Drawing for the job (mm, zero at the part's lowest x, y, z). Give positions to 0.01 mm unless a question says otherwise; leave off trailing zeros. Loops run counter-clockwise (first coordinate to the right, second up) from the corner with the lowest first, then second, coordinate; pieces in that order, holes last. Notation, with made-up numbers: (58, -8.75) -> (64, -8.75) arc R17 ccw to (64, 14.25) -> close; hole circle Ø4 at (44, 58). An arc over 180 degrees is marked (long way). Use CSV: the item, a comma, the result in double quotes. Start each with the question number.
(1) Cut at A-A on y = 5. Write the cut outline in (x, z).
(2) Flat gauge pins, fed straight in: pin 1 (1 mm diameter, centred on x = 33, y = 20, fed in from +Z); pin 2 (5 mm diameter, centred on y = 30, z = 51, fed in from +X); pin 3 (8 mm diameter, centred on y = 22, z = 18, fed in from +X). Where does each tip first touch, or does it go through?
(3) Pull direction Z, two halves, no side cores. Call the marked faces 1, 2, 3 and 4: pulls with the +Z half, pulls with the -Z half, needs draft (parallel to the pull), parting line crosses it, or undercut.
(4) Cut at C-C on z = 36. Write the cut outline in (x, y).
(5) Cut at B-B on x = 36. Write the cut outline in (y, z).
(6) Drill centre lines: probe 1 along Z at (x, y) = (35, 19); probe 2 along Z at (x, y) = (60, 4); probe 3 along X at (y, z) = (30.5, 52.5). Where is each one in solid material? Low to high.
(7) Cut at D-D on y = 26. Write the cut outline in (x, z).
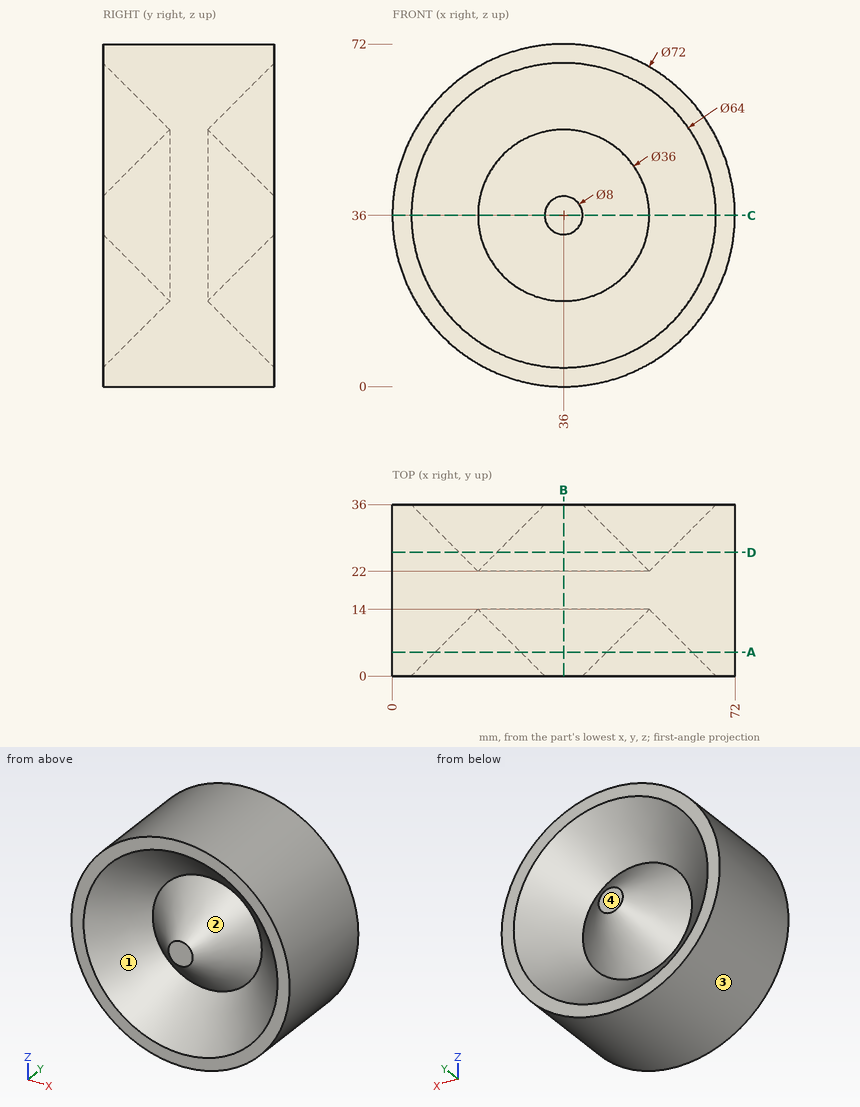
Check result:
1,outline,"circle Ø72 at (36, 36); circle Ø18 at (36, 36); hole circle Ø54 at (36, 36)"
2,pin 1,"z = 71.91"
2,pin 2,"x = 69.76"
2,pin 3,"x = 69.17"
3,face 1,"undercut"
3,face 2,"undercut"
3,face 3,"parting line crosses it"
3,face 4,"needs draft"
4,outline,"(0, 0) -> (4, 0) -> (18, 14) -> (32, 0) -> (40, 0) -> (54, 14) -> (68, 0) -> (72, 0) -> (72, 36) -> (68, 36) -> (54, 22) -> (40, 36) -> (32, 36) -> (18, 22) -> (4, 36) -> (0, 36) -> close"
5,outline,"(0, 0) -> (36, 0) -> (36, 4) -> (22, 18) -> (36, 32) -> (36, 40) -> (22, 54) -> (36, 68) -> (36, 72) -> (0, 72) -> (0, 68) -> (14, 54) -> (0, 40) -> (0, 32) -> (14, 18) -> (0, 4) -> close"
6,probe 1,"0.01 to 71.99"
6,probe 2,"9.17 to 21.58, 50.42 to 62.83"
6,probe 3,"4 to 15.26, 56.74 to 68"
7,outline,"circle Ø72 at (36, 36); circle Ø28 at (36, 36); hole circle Ø44 at (36, 36)"
